from build123d import *

# Parameters (mm, degrees)
F1_DEPTH = 2
F3_DEPTH = 2.1
F5_DEPTH = 2
F6_R     = 4


with BuildPart() as f1:
    # F0 (on Front) → F1 (new body)
    with BuildSketch(Plane.XZ):
        Polygon((-118.5, 62), (-118.5, 0), (-111.5, 0), (-111.5, 55), (111.5, 55), (111.5, 0), (118.5, 0), (118.5, 62), align=None)
    extrude(amount=F1_DEPTH)

    # F2 (on face) → F3 (join)
    with BuildSketch(Plane.XZ.offset(2)):
        Polygon((-118.5, 62), (-118.5, 0), (-116.6, 0), (-116.6, 59.4), (116.6, 59.4), (116.6, 0), (118.5, 0), (118.5, 62), align=None)
    extrude(amount=F3_DEPTH)

    # F4 (on face) → F5 (join)
    with BuildSketch(Plane.XZ.offset(4.1)):
        Polygon((-118.5, 62), (-118.5, 0), (-111.5, 0), (-111.5, 55), (111.5, 55), (111.5, 0), (118.5, 0), (118.5, 62), align=None)
    extrude(amount=F5_DEPTH)

    # F6
    f6_edges = [f1.edges().sort_by_distance(p)[0] for p in [
        (-118.5, -3.05, 62),
        (118.5, -3.05, 62),
    ]]
    fillet(f6_edges, radius=F6_R)


solid = f1.part
Verification items for the finished model (mm, model axes). A direction names the side the tool comes from. Coordinates: 2 decimals unless noted, no trailing zeros. Write each loop counter-clockwise with the first axis right and the second up, starting at its lowest first coordinate (ties: lowest second). Pieces come first, ordered by that corner, then holes. Notation, with made-up numbers: M -26,71 L 10,71 A25 cw 10,104 Z; hole C 86,59.5 d3. An arc over 180 degrees is marked long. One line per question, with ' | ' between items.
1) Material ranges on L1, parallel to X at y = -4, z = 16.5; L2, parallel to X at y = -5.25, z = 53; L3, parallel to Z at x = -100, y = -2.5, recorded low to high.
Solutions:
L1: -118.5 to -116.6, 116.6 to 118.5 | L2: -118.5 to -111.5, 111.5 to 118.5 | L3: 59.4 to 62
2) Sectioned sample at B-B on x = 102. Record the cut outline in (y, z), then the cut area to 3 significant figures.
Solutions:
outline: M -6.1,55 L -4.1,55 L -4.1,59.4 L -2,59.4 L -2,55 L 0,55 L 0,62 L -6.1,62 Z | area: 33.5 mm^2
3) Access from +Z, -Z, +X, -X, +Y, -Y to the whole of each face (thin tool, end or side, straight path). Record for faces 1 (the face through (-9, -2, 56)), 2 (the face through (-117.359, -3.007, 60.797)).
Solutions:
face 1: -Z | face 2: +Z, -X, +Y, -Y
4) Depth check by flat-ended pin: pin 1 Ø3 at (x, z) = (-36.5, 53) entering from -Y; pin 2 Ø3 at (x, y) = (-17, -5) entering from -Z. Enter the tip coordinate at first touch or a pass-through.
Solutions:
pin 1: through | pin 2: z = 55
5) Release check for a two-part mould opening along X. For faces 3 (the face through (-9, -4.1, 56)), 4 (the face through (117.359, -3.007, 60.797)), 5 (the face through (-117, -3, 0)) record: +X half, -X half, draft (parallel to the pull), parting line (faces both ways), or undercut.
Solutions:
face 3: undercut | face 4: +X half | face 5: draft
6) Sectioned sample at A-A on z = 15. Record the cut outline in (x, y), then the cut area to 3 significant figures.
Solutions:
outline: M -118.5,-6.1 L -111.5,-6.1 L -111.5,-4.1 L -116.6,-4.1 L -116.6,-2 L -111.5,-2 L -111.5,0 L -118.5,0 Z; M 111.5,-6.1 L 118.5,-6.1 L 118.5,0 L 111.5,0 L 111.5,-2 L 116.6,-2 L 116.6,-4.1 L 111.5,-4.1 Z | area: 64.0 mm^2
